from build123d import *

# Parameters (mm, degrees)
F_9_32_0_28125_DIAMETER_HOLE1_D   = 7.14375
PIPE_TAP_DRILL_FOR_1_8_TAP2_D     = 8.4328
PIPE_TAP_DRILL_FOR_1_8_TAP2_DEPTH = 12.7
PIPE_TAP_DRILL_FOR_1_8_TAP2_TIP   = 2.533468714


with BuildPart() as part:
    # Sketch1 → Revolve1 (revolve)
    with BuildSketch(Plane.XY, mode=Mode.PRIVATE) as revolve1_sk:
        Polygon((0, 0), (0, 6.731), (19.05, 6.731), (19.05, 9.525), (22.225, 9.525), (22.225, 0), align=None)
    revolve(revolve1_sk.sketch.rotate(Axis((0, 0, 0), (1, 0, 0)), 90), axis=Axis((0, 0, 0), (1, 0, 0)))

    # 9/32 (0.28125) Diameter Hole1 (through all)
    with Locations(Plane(origin=(22.225, 0, 0), x_dir=(0, 0, -1), z_dir=(1, 0, 0))):
        with Locations((0, 0)):
            Hole(F_9_32_0_28125_DIAMETER_HOLE1_D / 2)

    # Pipe Tap Drill for 1/8 Tap2
    with Locations(Plane.ZY):
        with Locations((0, 0)):
            Hole(PIPE_TAP_DRILL_FOR_1_8_TAP2_D / 2, depth=PIPE_TAP_DRILL_FOR_1_8_TAP2_DEPTH)
            with Locations((0, 0, -(PIPE_TAP_DRILL_FOR_1_8_TAP2_DEPTH + PIPE_TAP_DRILL_FOR_1_8_TAP2_TIP / 2))):  # 118° drill point
                Cone(0, PIPE_TAP_DRILL_FOR_1_8_TAP2_D / 2, PIPE_TAP_DRILL_FOR_1_8_TAP2_TIP, mode=Mode.SUBTRACT)


solid = part.part
Design review of the part built by this model. Coordinates are the model's own, in mm. A direction names the side the tool comes from. Give positions to 0.01 mm unless a question says otherwise; leave off trailing zeros. Loops run counter-clockwise (first coordinate to the right, second up) from the corner with the lowest first, then second, coordinate; pieces in that order, holes last. Notation, with made-up numbers: (-19.75, 52.25) -> (-9.75, 52.25) arc R18 ccw to (-9.75, 61.25) -> close; hole circle Ø2 at (-7, -34). An arc over 180 degrees is marked (long way). One line per question, with ' | ' between items. Start each with the question number.
(1) We need section A-A (y = 0). State the section outline as (x, z) points (3 decimals), and give its area (3 significant figures).
(2) For line 1 (Y direction, x = 19, z = 0); line 2 (Y direction, x = 19.75, z = 0) (3 decimals); line 3 (X direction, y = -6, z = -6.5) (3 decimals), list the stretches that pass through material, from the lowest coordinate up.
(3) We need section C-C (x = 10). State the section outline as (y, z) points.
(4) For faces 5 (the face through (9.66, 5.97, 3.11)), 6 (the face through (0, 4.4, 0.1)), list the 3-axis set-ups (+Z, -Z, +X, -X, +Y, -Y) from which the entire face can be reached by the end or side of a thin tool; tool diameter is ignored.
(5) Insertion check: P1, Ø5, axis at x = 17, z = -4.5, coming from the -Y side; P2, Ø5, axis at y = 0, z = 0, coming from the +X side; P3, Ø4, axis at x = 15.5, y = -3.5, coming from the +Z side; P4, Ø1, axis at x = 18.5, y = -3.5, coming from the +Z side. Each pin has a flat end and moves straight along its axis. Give the tip position at first contact, or say it passes through.
(6) Draft analysis for pull direction Y (two halves, no side actions). For faces 1 (the face through (19.05, -2.3, 6.5)), 2 (the face through (17.6, 1.1, 3.4)), 3 (the face through (6.44, 4.18, 0.55)), 4 (the face through (20.66, 9.3, -2.06)), state which applies: +Y half, -Y half, draft (parallel to the pull), parting line (faces both ways), or undercut.
(7) We need section D-D (z = -5.25). State the section outline as (x, y) points (3 decimals).
The answers:
1) outline: (0, -6.731) -> (19.05, -6.731) -> (19.05, -9.525) -> (22.225, -9.525) -> (22.225, -3.572) -> (13.087, -3.572) -> (12.7, -4.216) -> (0, -4.216) -> close; (0, 4.216) -> (12.7, 4.216) -> (13.087, 3.572) -> (22.225, 3.572) -> (22.225, 9.525) -> (19.05, 9.525) -> (19.05, 6.731) -> (0, 6.731) -> close | area: 142 mm^2
2) line 1: y = -6.73 to -3.57, 3.57 to 6.73 | line 2: y = -9.525 to -3.572, 3.572 to 9.525 | line 3: x = 19.05 to 22.225
3) outline: circle Ø13.46 at (0, 0); hole circle Ø8.43 at (0, 0)
4) face 5: -X | face 6: +Z, -Z, -X, +Y, -Y
5) P1: stops at y = -9.02 | P2: passes through | P3: stops at z = 6.56 | P4: stops at z = 6.03
6) face 1: draft | face 2: undercut | face 3: undercut | face 4: parting line
7) outline: (0, -4.212) -> (19.05, -4.212) -> (19.05, -7.948) -> (22.225, -7.948) -> (22.225, 7.948) -> (19.05, 7.948) -> (19.05, 4.212) -> (0, 4.212) -> close
